from build123d import *

# Parameters (mm, degrees)
F0_R     = 4.7625
F1_DEPTH = 25.4
F2_R     = 3.175
F3_DEPTH = 19.05
F5_DEPTH = 3.175


with BuildPart() as f1:
    # F0 (on Front) → F1 (new body)
    with BuildSketch(Plane.XZ):
        Circle(F0_R)
    extrude(amount=F1_DEPTH)

    # F2 (on face) → F3 (cut)
    with BuildSketch(Plane.XZ.offset(25.4)):
        Circle(F2_R)
    extrude(amount=-F3_DEPTH, mode=Mode.SUBTRACT)

    # F4 (on face) → F5 (join)
    with BuildSketch(Plane.XZ.offset(25.4)):
        with BuildLine():
            ThreePointArc((0, -4.7625), (-4.7625, 0), (0, 4.7625))
            Line((0, 4.7625), (-12.7, 4.7625))
            ThreePointArc((-12.7, 4.7625), (-13.5980256121, 4.3905256121), (-13.97, 3.4925))
            Line((-13.97, 3.4925), (-13.97, -3.4925))
            ThreePointArc((-13.97, -3.4925), (-13.5980256121, -4.3905256121), (-12.7, -4.7625))
            Line((-12.7, -4.7625), (0, -4.7625))
        make_face()
        with BuildLine():
            Line((12.7, 4.7625), (0, 4.7625))
            ThreePointArc((0, 4.7625), (3.3675960454, 3.3675960454), (4.7625, 0))
            ThreePointArc((4.7625, 0), (3.3675960454, -3.3675960454), (0, -4.7625))
            Line((0, -4.7625), (12.7, -4.7625))
            ThreePointArc((12.7, -4.7625), (13.5980256121, -4.3905256121), (13.97, -3.4925))
            Line((13.97, -3.4925), (13.97, 3.4925))
            ThreePointArc((13.97, 3.4925), (13.5980256121, 4.3905256121), (12.7, 4.7625))
        make_face()
    extrude(amount=-F5_DEPTH)


solid = f1.part
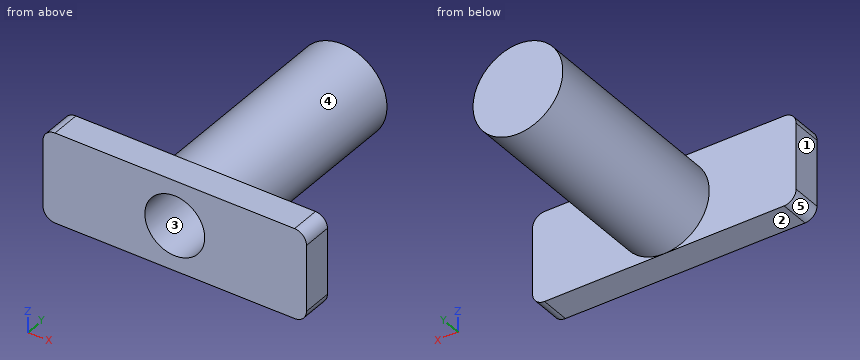
Input: part model. Units: mm. Frame: model coordinates. Face numbers are marked on the shaded views. A direction names the side the tool comes from. Give positions to 0.01 mm unless a question says otherwise; leave off trailing zeros. Write each loop counter-clockwise with the first axis right and the second up, starting at its lowest first coordinate (ties: lowest second). Pieces come first, ordered by that corner, then holes.
Q1. First-contact query: P1, Ø3, axis at x = 0, z = -1.5, coming from the -Y side; P2, Ø3, axis at x = 7.5, z = 0.5, coming from the +Y side (3 decimals); P3, Ø2, axis at y = -18.5, z = 3.5, coming from the +X side. Flat tips, straight axial feed; report the tip coordinate or a pass-through.
Q2. Material intervals for probe 1 along Z at (x, y) = (0, -15.75) (1 decimal); probe 2 along Y at (x, z) = (10, -2.25) (3 decimals); probe 3 along X at (y, z) = (-9.75, -1.5), sorted ascending.
Q3. Pull-direction query (Z, two-part tool) for the marked faces 1, 2 and 3; classes: pulls with the +Z half, pulls with the -Z half, needs draft (parallel to the pull), parting line crosses it, or undercut.
Q4. Section B-B, the plane x = -11. Output: boundary loops of the cut face in (y, z) (1 decimal), plus the area to 3 significant figures.
Q5. Set-up query: the marked faces 4 and 5. Return all of +Z, -Z, +X, -X, +Y, -Y with unobstructed straight access to the full face (end or side cutting, diameter ignored); none if empty.
Q6. Section D-D, the plane z = -1.75. Output: boundary loops of the cut face in (x, y) (3 decimals), plus the area to 3 significant figures.
Filled in:
1. P1: stops at y = -6.35
1. P2: stops at y = -22.225
1. P3: stops at x = 4.05
2. probe 1: z = -4.8 to -3.2, 3.2 to 4.8
2. probe 2: y = -25.4 to -22.225
2. probe 3: x = -4.52 to -2.8, 2.8 to 4.52
3. face 1: needs draft
3. face 2: pulls with the -Z half
3. face 3: undercut
4. outline: (-25.4, -4.8) - (-22.2, -4.8) - (-22.2, 4.8) - (-25.4, 4.8) - close
4. area: 30.2 mm2
5. face 4: +Y
5. face 5: -Z, -X, +Y, -Y
6. outline: (-13.97, -25.4) - (-2.649, -25.4) - (-2.649, -6.35) - (2.649, -6.35) - (2.649, -25.4) - (13.97, -25.4) - (13.97, -22.225) - (4.429, -22.225) - (4.429, 0) - (-4.429, 0) - (-4.429, -22.225) - (-13.97, -22.225) - close
6. area: 185 mm2
